Could you check a few things on this drawing? It's one solid part, dimensions in mm from its lowest x, y, z. A direction names the side the tool comes from. Round coordinates to 2 decimals unless told otherwise and drop trailing zeros. Loops run counter-clockwise (first coordinate to the right, second up) from the corner with the lowest first, then second, coordinate; pieces in that order, holes last. Notation, with made-up numbers: (51.25, 19) -> (76.25, 19) arc R26 cw to (76.25, 46) -> close; hole circle Ø5 at (-30, 69.5). An arc over 180 degrees is marked (long way). Write each question's results on one line, items separated by ' | '.
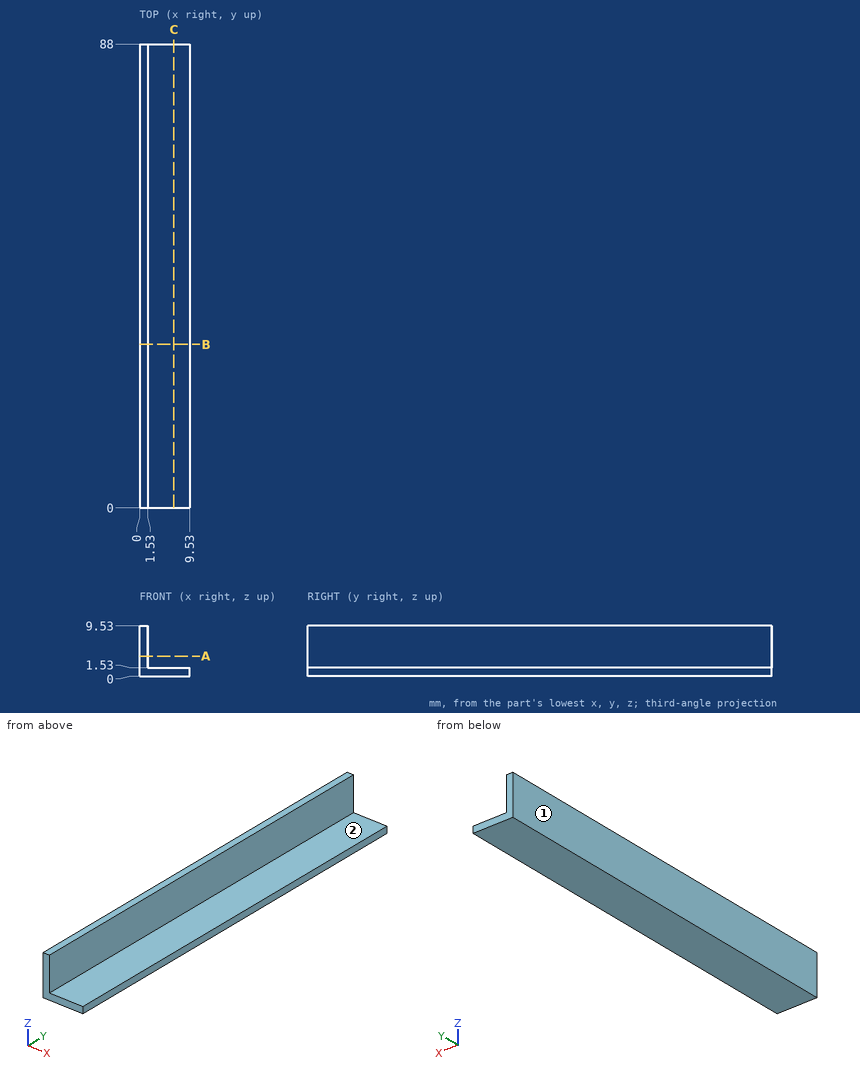
1) For the marked faces 1 and 2, which set-ups out of +Z, -Z, +X, -X, +Y, -Y let a thin tool reach every point of the face, with its end or its side?
Model answer:
face 1: +Z, -Z, -X, +Y, -Y | face 2: +Z, +X, +Y, -Y
2) I want a section at A-A, the plane z = 3.75. Write out the boundary of the cut face in (x, y).
Model answer:
outline: (0, 0) -> (1.53, 0) -> (1.53, 88) -> (0, 88) -> close
3) I want a section at B-B, the plane y = 31. Write out the boundary of the cut face in (x, z).
Model answer:
outline: (0, 0) -> (9.53, 0) -> (9.53, 1.53) -> (1.53, 1.53) -> (1.53, 9.53) -> (0, 9.53) -> close
4) I need wall thicknesses on line 1 (X direction, y = 37.5, z = 3.75). Which ranges of the line are inside material? Lowest first, please.
Model answer:
line 1: x = 0 to 1.53
5) I want a section at C-C, the plane x = 6.5. Write out the boundary of the cut face in (y, z), plus the area to 3 significant figures.
Model answer:
outline: (0, 0) -> (88, 0) -> (88, 1.53) -> (0, 1.53) -> close | area: 135 mm2
6) I'm going to push flat-ended pins straight in: pin 1 (1 mm diameter, centred on x = 8, z = 3.5, fed in from -Y); pin 2 (2.5 mm diameter, centred on x = 4.5, y = 58, fed in from +Z). Where does each tip first touch, or does it pass through?
Model answer:
pin 1: passes through | pin 2: stops at z = 1.53
